Geometry: final body of the model. Coordinates: model frame, mm. A direction names the side the tool comes from. Coordinates: 2 decimals unless noted, no trailing zeros. Write each loop counter-clockwise with the first axis right and the second up, starting at its lowest first coordinate (ties: lowest second). Pieces come first, ordered by that corner, then holes. Notation, with made-up numbers: M 3.5,-13 L 11.5,-13 A11 ccw 11.5,1 Z; hole C 17,14 d9. An arc over 180 degrees is marked long. Write item = value, one per line. Start each with the question number.
Item 1: Section D-D on x = 0.8. Output: boundary loops of the cut face in (y, z).
Item 2: Section A-A on x = -0.85. Output: boundary loops of the cut face in (y, z), plus the area to 3 significant figures.
Item 3: Ray query, L1, parallel to Y at x = -1.15, z = -7.75; L2, parallel to Z at x = -0.15, y = -1.05; L3, parallel to Z at x = 1.05, y = -2. Return the intervals inside material, ascending. Write a range as [from, to].
Item 4: Section C-C on z = 1.25. Output: boundary loops of the cut face in (x, y) (3 decimals).
Item 5: Reachability of faces 1 (the flat face through (0, -2.54, 15)), 2 (the cylindrical face through (0.88, -0.53, 16.93)) from +Z, -Z, +X, -X, +Y, -Y: full face, straight path, thin tool, end or side. Return the list, or none.
Item 6: Section B-B on y = 1.65. Output: boundary loops of the cut face in (x, z) (3 decimals).
Item 7: First-contact query: pin 1 Ø1.5 at (x, y) = (-1, 1) entering from +Z; pin 2 Ø1 at (x, z) = (0.5, -2) entering from -Y. Flat tips, straight axial feed; report the tip coordinate or a pass-through.
from build123d import *

# Parameters (mm, degrees)
BOSS_EXTRUDE1_DEPTH = 2.54
BOSS_EXTRUDE2_DEPTH = 2.54


with BuildPart() as part:
    # Sketch1 → Boss-Extrude1 (new body)
    with BuildSketch(Plane(origin=(0, 0, 0), x_dir=(1, 0, 0), z_dir=(0, 1, 0))):
        with BuildLine():
            ThreePointArc((-1.905, 2.54), (0, 3.175), (1.905, 2.54))
            Line((1.905, 2.54), (1.905, 10.16))
            ThreePointArc((1.905, 10.16), (0, 12.065), (-1.905, 10.16))
            Line((-1.905, 10.16), (-1.905, 2.54))
        make_face()
        with BuildLine():
            Line((1.905, -15.24), (1.905, 2.54))
            ThreePointArc((1.905, 2.54), (0, 3.175), (-1.905, 2.54))
            Line((-1.905, 2.54), (-1.905, -15.24))
            ThreePointArc((-1.905, -15.24), (0, -13.335), (1.905, -15.24))
        make_face()
    extrude(amount=BOSS_EXTRUDE1_DEPTH)

    # Sketch1_3 → Boss-Extrude2 (add, symmetric)
    with BuildSketch(Plane(origin=(0, 0, 0), x_dir=(1, 0, 0), z_dir=(0, 1, 0))):
        with BuildLine():
            ThreePointArc((-1.905, -15.24), (0, -17.145), (1.905, -15.24))
            ThreePointArc((1.905, -15.24), (0, -13.335), (-1.905, -15.24))
        make_face()
    extrude(amount=BOSS_EXTRUDE2_DEPTH, both=True)


solid = part.part
Responses:
q1.outline = M -2.54,13.51 L 0,13.51 L 0,-11.89 L 2.54,-11.89 L 2.54,16.97 L -2.54,16.97 Z
q2.outline = M -2.54,13.54 L 0,13.54 L 0,-11.86 L 2.54,-11.86 L 2.54,16.94 L -2.54,16.94 Z
q2.area = 81.8 mm²
q3.L1 = [0, 2.54]
q3.L2 = [13.34, 17.14]
q3.L3 = [13.65, 16.83]
q4.outline = M -1.905,0 L 1.905,0 L 1.905,2.54 L -1.905,2.54 Z
q5.face_1 = +Z, -Z, +X, -X, -Y
q5.face_2 = -Y
q6.outline = M -1.905,-10.16 A1.905 ccw 1.905,-10.16 L 1.905,15.24 A1.905 ccw -1.905,15.24 Z
q7.pin_1 = 17.13
q7.pin_2 = 0
